Could you check a few things on this model? Use its own coordinates, in mm. Face numbers are marked on the shaded views. A direction names the side the tool comes from. Round coordinates to 2 decimals unless told otherwise and drop trailing zeros. Loops run counter-clockwise (first coordinate to the right, second up) from the corner with the lowest first, then second, coordinate; pieces in that order, holes last. Notation, with made-up numbers: M -19,-30.5 L 10,-30.5 A24 cw 10,8.5 Z; hole C 33,39 d2. An arc over 180 degrees is marked long. Return JSON: item names as keys, results as strings. Group by question number.
```python
from build123d import *

# Parameters (mm, degrees)
F2_DEPTH = 600
F1_W     = 600
F1_H     = 380
F3_DEPTH = 18
F4_W     = 564
F4_H     = 377
F5_DEPTH = 18


with BuildPart() as f2:
    # F0 (on Top) → F2 (new body)
    with BuildSketch(Plane.XY):
        Polygon((81.165642, 334.102758), (-518.834358, 334.102758), (-518.834358, -45.897242), (-500.834358, -45.897242), (-500.834358, 331.102758), (63.165642, 331.102758), (63.165642, -45.897242), (81.165642, -45.897242), align=None)
    extrude(amount=F2_DEPTH)

    # F1 (on Top) → F3 (join)
    with BuildSketch(Plane.XY):
        with Locations((-218.834358, 144.102758)):
            Rectangle(F1_W, F1_H)
    extrude(amount=F3_DEPTH)

    # F4 (on face) → F5 (join)
    with BuildSketch(Plane.XY.offset(600)):
        with Locations((-218.834358, 142.602758)):
            Rectangle(F4_W, F4_H)
    extrude(amount=-F5_DEPTH)


solid = f2.part
```
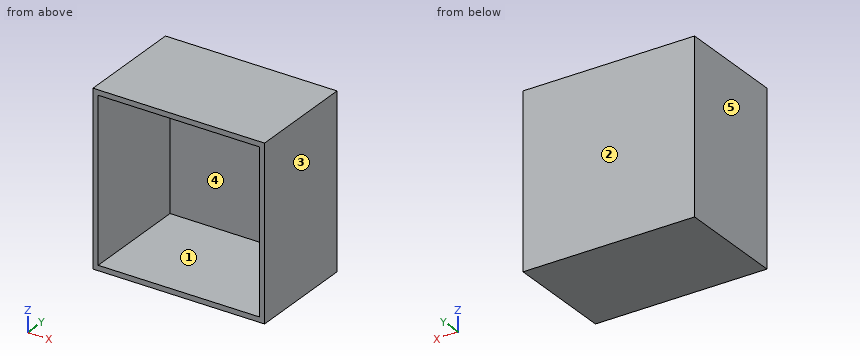
1. On a 3-axis mill with a long thin cutter (end or side, diameter ignored), from which of +Z, -Z, +X, -X, +Y, -Y can I reach the whole of each face in a straight line? I mean the marked faces 4 and 5. Say none if no direction works.
2. If we section it at A-A, the plane y = 176.5: Please give me the cut outline in (x, z).
3. If we section it at C-C, the plane z = 250: Please give me the cut outline in (x, y).
4. If we section it at B-B, the plane x = -389: Please give me the cut outline in (y, z).
5. We'd pull the mould along X, two halves only. Please class the marked faces 1, 2 and 3: +X half, -X half, draft (parallel to the pull), parting line (faces both ways), or undercut.
6. I need wall thicknesses on probe 1 along X at (y, z) = (198, 83); probe 2 along Z at (x, y) = (-480, 128); probe 3 along Y at (x, z) = (-393.5, 550). Which ranges of each line are inside material? Lowest first, please.
Geometry results:
{
 "1": {"face 4": "-Y", "face 5": "+Z, -Z, -X, +Y, -Y"},
 "2": {"outline": "M -518.83,0 L 81.17,0 L 81.17,600 L -518.83,600 Z; hole M -500.83,18 L 63.17,18 L 63.17,582 L -500.83,582 Z"},
 "3": {"outline": "M -518.83,-45.9 L -500.83,-45.9 L -500.83,331.1 L 63.17,331.1 L 63.17,-45.9 L 81.17,-45.9 L 81.17,334.1 L -518.83,334.1 Z"},
 "4": {"outline": "M -45.9,0 L 334.1,0 L 334.1,600 L -45.9,600 L -45.9,582 L 331.1,582 L 331.1,18 L -45.9,18 Z"},
 "5": {"face 1": "undercut", "face 2": "draft", "face 3": "+X half"},
 "6": {"probe 1": "-518.83 to -500.83, 63.17 to 81.17", "probe 2": "0 to 18, 582 to 600", "probe 3": "331.1 to 334.1"}
}
